```python
from build123d import *

# Parameters (mm, degrees)
BOSS_EXTRUDE1_DEPTH   = 22.225
CUT_EXTRUDE1_REACH    = 12.357
FILLET1_R             = 2.54
F_4_CLEARANCE_HOLE1_D = 3.4544
SKETCH6_W             = 5.1625
SKETCH6_H             = 1.9875
CUT_EXTRUDE2_DEPTH    = 8.255


with BuildPart() as part:
    # Sketch1 → Boss-Extrude1 (new body)
    with BuildSketch(Plane.XY):
        Polygon((-96.82388635, -119.84135975), (-47.294090685, -119.983632078), (-47.323432737, -130.198589936), (-60.023380343, -130.162109852), (-60.005140301, -123.812136049), (-84.135040753, -123.742823889), (-84.153280795, -130.092797692), (-96.853228402, -130.056317608), align=None)
    extrude(amount=BOSS_EXTRUDE1_DEPTH)

    # Sketch2 → Cut-Extrude1 (cut, up to next)
    with BuildSketch(Plane(origin=(-0.345035492, -120.118491334, 0), x_dir=(0.999995875, -0.002872448, 0), z_dir=(0.002872448, 0.999995875, 0)), mode=Mode.PRIVATE) as cut_extrude1_sk1:
        with BuildLine():
            Line((-67.837073069, -4.8775), (-75.591424695, -4.8775))
            ThreePointArc((-75.591424695, -4.8775), (-71.714248882, -18.4546875), (-67.837073069, -4.8775))
        make_face()
    cut_extrude1_tool1 = extrude(cut_extrude1_sk1.sketch, amount=-CUT_EXTRUDE1_REACH, mode=Mode.PRIVATE) & part.part
    add(cut_extrude1_tool1.solids().sort_by_distance((-72.058989, -119.912496, 11.350092))[0], mode=Mode.SUBTRACT)

    # Fillet1
    fillet1_edges = [part.edges().sort_by_distance(p)[0] for p in [
        (-96.82388635, -119.84135975, 11.1125),
        (-47.294090685, -119.983632078, 11.1125),
        (-47.323432737, -130.198589936, 11.1125),
        (-60.023380343, -130.162109852, 11.1125),
        (-60.005140301, -123.812136049, 11.1125),
        (-84.135040753, -123.742823889, 11.1125),
        (-84.153280795, -130.092797692, 11.1125),
        (-96.853228402, -130.056317608, 11.1125),
    ]]
    fillet(fillet1_edges, radius=FILLET1_R)

    # #4 Clearance Hole1 (through all)
    with Locations(Plane.XY.offset(22.225)):
        with Locations((-90.488583573, -124.967078721), (-53.658735514, -125.072870965)):
            Hole(F_4_CLEARANCE_HOLE1_D / 2)

    # Sketch6 → Cut-Extrude2 (cut)
    with BuildSketch(Plane(origin=(-0.345035492, -120.118491334, 0), x_dir=(0.999995875, -0.002872448, 0), z_dir=(0.002872448, 0.999995875, 0))):
        with Locations((-90.129248882, -16.35125)):
            Rectangle(SKETCH6_W, SKETCH6_H)
        with Locations((-90.129248882, -5.87375)):
            Rectangle(SKETCH6_W, SKETCH6_H)
        with Locations((-53.299248882, -5.87375)):
            Rectangle(SKETCH6_W, SKETCH6_H)
        with Locations((-53.299248882, -16.35125)):
            Rectangle(SKETCH6_W, SKETCH6_H)
    extrude(amount=-CUT_EXTRUDE2_DEPTH, mode=Mode.SUBTRACT)


solid = part.part
```
Read the model definition and answer for the solid it produces. Units are mm, in the model's axes. Coordinates: 2 decimals unless noted, no trailing zeros. Loops run counter-clockwise (first coordinate to the right, second up) from the corner with the lowest first, then second, coordinate; pieces in that order, holes last. Notation, with made-up numbers: (24, 9.5) -> (41, 9.5) arc R12 cw to (41, 31.5) -> close; hole circle Ø2 at (21, 28.5). An arc over 180 degrees is marked (long way). Return JSON: item names as keys, results as strings.
Item 1: Find section B-B (z = 16.25). Determine the outline of the cut face in (x, y), plus the area to 3 significant figures.
Answers:
{"outline": "(-96.85, -127.52) arc R2.54 ccw to (-94.31, -130.06) -> (-86.69, -130.09) arc R2.54 ccw to (-84.15, -127.55) -> (-84.14, -126.28) arc R2.54 cw to (-81.6, -123.75) -> (-77.32, -123.76) -> (-77.3, -119.9) -> (-87.89, -119.87) -> (-87.92, -128.12) -> (-93.08, -128.11) -> (-93.06, -119.85) -> (-94.28, -119.85) arc R2.54 ccw to (-96.83, -122.38) -> close; (-66.82, -123.79) -> (-62.55, -123.8) arc R2.54 cw to (-60.01, -126.35) -> (-60.02, -127.62) arc R2.54 ccw to (-57.48, -130.17) -> (-49.86, -130.19) arc R2.54 ccw to (-47.32, -127.66) -> (-47.3, -122.52) arc R2.54 ccw to (-49.83, -119.98) -> (-51.06, -119.97) -> (-51.09, -128.23) -> (-56.25, -128.21) -> (-56.23, -119.96) -> (-66.81, -119.93) -> close", "area": "221 mm2"}
Item 2: Find section C-C (z = 19.25). Determine the outline of the cut face in (x, y).
Answers:
{"outline": "(-96.85, -127.52) arc R2.54 ccw to (-94.31, -130.06) -> (-86.69, -130.09) arc R2.54 ccw to (-84.15, -127.55) -> (-84.14, -126.28) arc R2.54 cw to (-81.6, -123.75) -> (-62.55, -123.8) arc R2.54 cw to (-60.01, -126.35) -> (-60.02, -127.62) arc R2.54 ccw to (-57.48, -130.17) -> (-49.86, -130.19) arc R2.54 ccw to (-47.32, -127.66) -> (-47.3, -122.52) arc R2.54 ccw to (-49.83, -119.98) -> (-94.28, -119.85) arc R2.54 ccw to (-96.83, -122.38) -> close; hole circle Ø3.45 at (-90.49, -124.97); hole circle Ø3.45 at (-53.66, -125.07)"}
Item 3: For a pull along Y with two mould halves and no side action, classify faces 1 (the cylindrical face through (-54.456, -126.605, 11.053)), 2 (the cylindrical face through (-91.4, -123.5, 2.4)) as +Y half, -Y half, draft (parallel to the pull), parting line (faces both ways), or undercut.
Answers:
{"face 1": "undercut", "face 2": "undercut"}
Item 4: Flat-ended cylindrical pins translate along their axes: P1, Ø4, axis at x = -61.5, z = 14, coming from the +Y side; P2, Ø2, axis at y = -125.5, z = 9, coming from the +X side; P3, Ø3, axis at x = -81.5, z = 6, coming from the -Y side. Find the tip coordinate at first contact, or state that the pin passes through.
Answers:
{"P1": "stops at y = -119.94", "P2": "stops at x = -47.31", "P3": "stops at y = -124.17"}
Item 5: Find section D-D (y = -120.75). Count the separate pieces of the cut face and the enclosed holes in it, plus the area to 3 significant figures.
Answers:
{"separate pieces": "1", "enclosed holes": "5", "area": "867 mm2"}
Item 6: Find section A-A (x = -91). Determine the outline of the cut face in (y, z) (1 decimal), plus the area to 3 significant figures.
Answers:
{"outline": "(-130.1, 0) -> (-126.6, 0) -> (-126.6, 4.9) -> (-128.1, 4.9) -> (-128.1, 6.9) -> (-126.6, 6.9) -> (-126.6, 15.4) -> (-128.1, 15.4) -> (-128.1, 17.3) -> (-126.6, 17.3) -> (-126.6, 22.2) -> (-130.1, 22.2) -> close; (-123.3, 0) -> (-119.9, 0) -> (-119.9, 4.9) -> (-123.3, 4.9) -> close; (-123.3, 6.9) -> (-119.9, 6.9) -> (-119.9, 15.4) -> (-123.3, 15.4) -> close; (-123.3, 17.3) -> (-119.9, 17.3) -> (-119.9, 22.2) -> (-123.3, 22.2) -> close", "area": "134 mm2"}
Item 7: Find the intervals of material crossed by probe 1 along Z at (x, y) = (-51.5, -122.75) (1 decimal); probe 2 along X at (y, z) = (-126, 17); probe 3 along X at (y, z) = (-125.25, 14.5), in increasing order.
Answers:
{"probe 1": "z = 0 to 4.9, 6.9 to 15.4, 17.3 to 22.2", "probe 2": "x = -96.84 to -93.07, -87.91 to -84.13, -60.04 to -56.24, -51.08 to -47.31", "probe 3": "x = -96.84 to -92.19, -88.78 to -83.92, -60.26 to -55.38, -51.94 to -47.31"}
